from build123d import *

# Parameters (mm, degrees)
F0_R     = 1.5
F1_DEPTH = 1.5


with BuildPart() as f1:
    # F0 (on Front) → F1 (new body)
    with BuildSketch(Plane.XZ):
        with BuildLine():
            ThreePointArc((0, 53.956001), (-27.215951, 46.589076), (-47, 26.5))
            Line((-47, 26.5), (-47, -26.5))
            ThreePointArc((-47, -26.5), (-27.215951, -46.589076), (0, -53.956001))
            ThreePointArc((0, -53.956001), (27.215951, -46.589076), (47, -26.5))
            Line((47, -26.5), (47, 26.5))
            ThreePointArc((47, 26.5), (27.215951, 46.589076), (0, 53.956001))
        make_face()
        with Locations((-42, -25)):
            Circle(F0_R, mode=Mode.SUBTRACT)
        with Locations((42, -25)):
            Circle(F0_R, mode=Mode.SUBTRACT)
        with Locations((-42, 25)):
            Circle(F0_R, mode=Mode.SUBTRACT)
        with BuildLine():
            ThreePointArc((-42, 19.8), (-37.01342, 23.525544), (-39.172119, 29.363839))
            ThreePointArc((-39.172119, 29.363839), (-21.899245, 43.784849), (0, 48.956))
            ThreePointArc((0, 48.956), (21.899245, 43.784849), (39.172119, 29.363839))
            ThreePointArc((39.172119, 29.363839), (37.01342, 23.525544), (42, 19.8))
            Line((42, 19.8), (42, -19.8))
            ThreePointArc((42, -19.8), (38.323045, -21.323045), (36.8, -25))
            Line((36.8, -25), (36.8, -30))
            Line((36.8, -30), (39.8, -30))
            Line((39.8, -30), (39.8, -32))
            Line((39.8, -32), (37.04983, -32))
            Line((37.04983, -32), (36.8, -32))
            Line((36.8, -32), (36.8, -32.286993))
            ThreePointArc((36.8, -32.286993), (20.199603, -44.594461), (0, -48.956))
            ThreePointArc((0, -48.956), (-20.199603, -44.594461), (-36.8, -32.286993))
            Line((-36.8, -32.286993), (-36.8, -32))
            Line((-36.8, -32), (-37.04983, -32))
            Line((-37.04983, -32), (-39.8, -32))
            Line((-39.8, -32), (-39.8, -30))
            Line((-39.8, -30), (-36.8, -30))
            Line((-36.8, -30), (-36.8, -25))
            ThreePointArc((-36.8, -25), (-38.323045, -21.323045), (-42, -19.8))
            Line((-42, -19.8), (-42, 19.8))
        make_face(mode=Mode.SUBTRACT)
        with Locations((42, 25)):
            Circle(F0_R, mode=Mode.SUBTRACT)
    extrude(amount=F1_DEPTH)


solid = f1.part
Design review of the part built by this model. Coordinates are the model's own, in mm. A direction names the side the tool comes from. Round coordinates to 2 decimals unless told otherwise and drop trailing zeros. Write each loop counter-clockwise with the first axis right and the second up, starting at its lowest first coordinate (ties: lowest second). Pieces come first, ordered by that corner, then holes. Notation, with made-up numbers: (45, 88) - (81, 88) arc R22 ccw to (81, 119) - close; hole circle Ø2 at (83, 51). An arc over 180 degrees is marked (long way). Return JSON: item names as keys, results as strings. Group by question number.
Item 1: For probe 1 along X at (y, z) = (-0.5, -6); probe 2 along X at (y, z) = (-0.4, 42.5); probe 3 along Z at (x, y) = (-27.5, -0.4), list the stretches that pass through material, from the lowest coordinate up. Write a range as [from, to].
Item 2: Machinability: for faces 1 (the face through (-39, 0, -24)), 2 (the face through (38.364, -0.74, -21.283)), which of the approach directions +Z, -Z, +X, -X, +Y, -Y give a long, thin tool a straight path to every point of the face, cutting with its end or side? Answer none if there is none.
Item 3: The part is to be moulded in two halves that separate along Z. For faces 3 (the face through (-43.11, -0.74, 26.01)), 4 (the face through (-37.04, -0.74, 23.44)), 5 (the face through (-39, -1.5, -24)), say which applies: pulls with the +Z half, pulls with the -Z half, needs draft (parallel to the pull), parting line crosses it, or undercut.
Item 4: We need section D-D on y = -0.85. Give the number of separate pieces and of enclosed holes in the cut face, and give its area (3 significant figures).
Item 5: We need section B-B on z = -9. Write out the cut boundary in (x, y).
Item 6: We need section C-C on x = 32. Write out the cut boundary in (y, z), and give its area (3 significant figures).
Item 7: We need section A-A on z = 25. Write out the cut boundary in (x, y).
Item 8: Insertion check: P1, Ø1.8, axis at x = 42, z = 25, coming from the +Y side; P2, Ø0.8, axis at y = -1, z = -31, coming from the -X side. Each pin has a flat end and moves straight along its axis. Give the tip position at first contact, or say it passes through.
Model answer:
{
 "1": {"probe 1": "x = [-47, -42], [42, 47]", "probe 2": "x = [-33.24, -24.3], [24.3, 33.24]", "probe 3": "z = [-46.42, -40.5], [40.5, 46.42]"},
 "2": {"face 1": "+Z, -Z, +X, -X, +Y", "face 2": "+Y, -Y"},
 "3": {"face 3": "undercut", "face 4": "undercut", "face 5": "needs draft"},
 "4": {"separate pieces": "1", "enclosed holes": "5", "area": "1,710 mm²"},
 "5": {"outline": "(-47, -1.5) - (-42, -1.5) - (-42, 0) - (-47, 0) - close; (42, -1.5) - (47, -1.5) - (47, 0) - (42, 0) - close"},
 "6": {"outline": "(-1.5, -43.44) - (0, -43.44) - (0, -37.05) - (-1.5, -37.05) - close; (-1.5, 37.05) - (0, 37.05) - (0, 43.44) - (-1.5, 43.44) - close", "area": "19.2 mm²"},
 "7": {"outline": "(-47, -1.5) - (-43.5, -1.5) - (-43.5, 0) - (-47, 0) - close; (-40.5, -1.5) - (-36.8, -1.5) - (-36.8, 0) - (-40.5, 0) - close; (36.8, -1.5) - (40.5, -1.5) - (40.5, 0) - (36.8, 0) - close; (43.5, -1.5) - (47, -1.5) - (47, 0) - (43.5, 0) - close"},
 "8": {"P1": "passes through", "P2": "stops at x = -44.44"}
}
